```python
from build123d import *

# Parameters (mm, degrees)
SKETCH2_R          = 1.5875
CUT_EXTRUDE1_DEPTH = 10.53
CIRPATTERN1_COUNT  = 3


with BuildPart() as part:
    # Sketch1 → Revolve1 (revolve)
    with BuildSketch(Plane.XY):
        Polygon((2.38, 9.53), (9.525, 9.53), (9.525, 6.35), (3.97, 6.35), (3.97, 0), (2.38, 0), align=None)
    revolve(axis=Axis((0, 10.340432257, 0), (0, -1, 0)))

    # Sketch2 → Cut-Extrude1 (cut, through all)
    with BuildSketch(Plane(origin=(0, 9.53, 0), x_dir=(1, 0, 0), z_dir=(0, 1, 0))):
        with Locations((0, 6.35)):
            Circle(SKETCH2_R)
    cut_extrude1 = extrude(amount=-CUT_EXTRUDE1_DEPTH, mode=Mode.SUBTRACT)

    # CirPattern1: Cut-Extrude1 ×3 about axis
    cirpattern1_axis = Axis((0, 0, 0), (0, 1, 0))
    for i in range(1, CIRPATTERN1_COUNT):
        add(cut_extrude1.rotate(cirpattern1_axis, i * 360 / CIRPATTERN1_COUNT), mode=Mode.SUBTRACT)


solid = part.part
```
Read the model definition and answer for the solid it produces. Units are mm, in the model's axes. A direction names the side the tool comes from. Give positions to 0.01 mm unless a question says otherwise; leave off trailing zeros. Loops run counter-clockwise (first coordinate to the right, second up) from the corner with the lowest first, then second, coordinate; pieces in that order, holes last.
Item 1: For faces 1 (the cylindrical face through (-3.985, 7.962, 2.698)), 2 (the cylindrical face through (3.787, 3.131, 1.192)), determine the directions among +Z, -Z, +X, -X, +Y, -Y from which every point of the face is accessible in a straight line to the end or side of a thin tool.
Item 2: The part is cut by section D-D (x = 5.25). Write down the section's boundary in (y, z).
Item 3: The mould has two halves that part along Z. Classify faces 3 (the cylindrical face through (0.73, 7.96, -4.94)), 4 (the flat face through (2, 0, -2)), 5 (the cylindrical face through (-7.559, 7.918, -5.796)): released by +Z, released by -Z, zero draft, split by the parting line, or undercut.
Item 4: The part is cut by section B-B (x = 0). Give the number of separate pieces and of enclosed holes in the cut face, and give its area (3 significant figures).
Item 5: The part is cut by section C-C (y = 6). Write down the section's boundary in (x, z), and give its area (3 significant figures).
Item 6: Each of these flat-tipped pins is pushed along its axis until it touches: pin 1 Ø3 at (x, y) = (1.5, 1) entering from -Z; pin 2 Ø1 at (x, y) = (5, 2.5) entering from +Z; pin 3 Ø3 at (y, z) = (3, -4) entering from -X. Where does it stop, or does it pass through?
Item 7: Find the intervals of material crossed by line 1 along Z through (x, y) = (0, 8.45) (1 decimal); line 2 along X through (y, z) = (7.5, 2.5); line 3 along Z through (x, y) = (0, 3), in increasing order.
Item 8: The part is cut by section A-A (z = 0). Write down the section's boundary in (x, y) (3 decimals).
Taken from the geometry:
1. face 1: +Y, -Y
1. face 2: -Y
2. outline: (6.35, -7.95) - (9.53, -7.95) - (9.53, 1.61) - (6.35, 1.61) - close; (6.35, 4.74) - (9.53, 4.74) - (9.53, 7.95) - (6.35, 7.95) - close
3. face 3: undercut
3. face 4: zero draft
3. face 5: split by the parting line
4. separate pieces: 3
4. enclosed holes: 0
4. area: 55.5 mm2
5. outline: circle Ø7.94 at (0, 0); hole circle Ø4.76 at (0, 0)
5. area: 31.7 mm2
6. pin 1: stops at z = -3.97
6. pin 2: passes through
6. pin 3: stops at x = -3.08
7. line 1: z = -9.5 to -7.9, -4.8 to -2.4, 2.4 to 9.5
7. line 2: x = -9.19 to -6.94, -4.06 to 4.06, 6.94 to 9.19
7. line 3: z = -3.97 to -2.38, 2.38 to 3.97
8. outline: (-9.525, 6.35) - (-3.97, 6.35) - (-3.97, 0) - (-2.38, 0) - (-2.38, 9.53) - (-9.525, 9.53) - close; (2.38, 0) - (3.97, 0) - (3.97, 6.35) - (9.525, 6.35) - (9.525, 9.53) - (2.38, 9.53) - close
